```python
from build123d import *

# Parameters (mm, degrees)
EXTRUDE_1_DEPTH           = 60
CUT_EXTRUDE_1_DEPTH       = 423.965719651
CUT_EXTRUDE_1_DEPTH_BACK  = 25
HOLE_WIZARD_1_D           = 20
HOLE_WIZARD_1_CBORE_D     = 40
HOLE_WIZARD_1_CBORE_DEPTH = 20
EXTRUDE_START             = -32
EXTRUDE_3_DEPTH           = 72
CUT_EXTRUDE_3_DEPTH       = 531.913363931
CUT_EXTRUDE_3_DEPTH_BACK  = 531.913363931
SKETCH_10_R               = 40
SKETCH_12_R               = 80
CUT_EXTRUDE_5_DEPTH       = 20


with BuildPart() as part:
    # 草图1 → 凸台-拉伸1 (new body)
    with BuildSketch(Plane(origin=(0, 0, 0), x_dir=(1, 0, 0), z_dir=(0, 1, 0))):
        with BuildLine():
            Line((0, 0), (288, 0))
            ThreePointArc((288, 0), (310.627416998, -9.372583002), (320, -32))
            Line((320, -32), (320, -238))
            ThreePointArc((320, -238), (310.627416998, -260.627416998), (288, -270))
            Line((288, -270), (0, -270))
            Line((0, -270), (0, 0))
        make_face()
    extrude(amount=EXTRUDE_1_DEPTH)

    # 草图2 → 切除-拉伸1 (cut, two sides: drawn at the far end of the back side and taken through both)
    with BuildSketch(Plane.XZ.offset(-CUT_EXTRUDE_1_DEPTH_BACK)):
        with BuildLine():
            Line((230, 195), (320, 195))
            Line((320, 195), (320, 75))
            Line((320, 75), (230, 75))
            ThreePointArc((230, 75), (170, 135), (230, 195))
        make_face()
    extrude(amount=CUT_EXTRUDE_1_DEPTH + CUT_EXTRUDE_1_DEPTH_BACK, mode=Mode.SUBTRACT)

    # 孔1 (through all)
    with Locations(Plane(origin=(0, 60, 0), x_dir=(1, 0, 0), z_dir=(0, 1, 0))):
        with Locations((230, -135)):
            CounterBoreHole(HOLE_WIZARD_1_D / 2, HOLE_WIZARD_1_CBORE_D / 2, HOLE_WIZARD_1_CBORE_DEPTH)

    # 草图8 → 凸台-拉伸3 (add)
    with BuildSketch(Plane.ZY.offset(EXTRUDE_START)):
        with BuildLine():
            Line((0, 60), (270, 60))
            Line((270, 60), (270, 220))
            ThreePointArc((270, 220), (135, 355), (0, 220))
            Line((0, 220), (0, 60))
        make_face()
    extrude(amount=-EXTRUDE_3_DEPTH)

    # 草图10 → 切除-拉伸3 (cut, two sides: drawn at the far end of the back side and taken through both)
    with BuildSketch(Plane.ZY.offset(-32).offset(-CUT_EXTRUDE_3_DEPTH_BACK)):
        with Locations((135, 220)):
            Circle(SKETCH_10_R)
    extrude(amount=CUT_EXTRUDE_3_DEPTH + CUT_EXTRUDE_3_DEPTH_BACK, mode=Mode.SUBTRACT)

    # 草图12 → 切除-拉伸5 (cut)
    with BuildSketch(Plane.ZY.offset(-32)):
        with BuildLine():
            Line((255, 60), (255, 220))
            ThreePointArc((255, 220), (135, 340), (15, 220))
            Line((15, 220), (15, 60))
            Line((15, 60), (255, 60))
        make_face()
        with Locations((135, 220)):
            Circle(SKETCH_12_R, mode=Mode.SUBTRACT)
    extrude(amount=-CUT_EXTRUDE_5_DEPTH, mode=Mode.SUBTRACT)


solid = part.part
```
Could you check a few things on this model? Use its own coordinates, in mm. A direction names the side the tool comes from. Round coordinates to 2 decimals unless told otherwise and drop trailing zeros. Loops run counter-clockwise (first coordinate to the right, second up) from the corner with the lowest first, then second, coordinate; pieces in that order, holes last. Notation, with made-up numbers: (76.25, 27.25) -> (126.25, 27.25) arc R24 ccw to (126.25, 51.25) -> close; hole circle Ø1 at (25, -5.5). An arc over 180 degrees is marked (long way). Put each result on its own line as item: value.
Q1. I want a section at A-A on z = 135. Write out the boundary of the cut face in (x, y), and give its area (3 significant figures).
Checks:
outline: (0, 0) -> (170, 0) -> (170, 25) -> (220, 25) -> (220, 40) -> (210, 40) -> (210, 60) -> (104, 60) -> (104, 180) -> (32, 180) -> (32, 140) -> (52, 140) -> (52, 60) -> (0, 60) -> close; (32, 260) -> (104, 260) -> (104, 355) -> (32, 355) -> (32, 340) -> (52, 340) -> (52, 300) -> (32, 300) -> close; (240, 25) -> (320, 25) -> (320, 60) -> (250, 60) -> (250, 40) -> (240, 40) -> close
area: 27,400 mm2
Q2. Thinking about a two-plate mould opening in Y: for faces 5 (the cylindrical face through (67.496, 354.967, 137.969)), 6 (the cylindrical face through (170.015, 12.675, 133.681)), 7 (the cylindrical face through (41.86, 339.97, 137.64)), which applies, pulls with the +Y half, pulls with the -Y half, needs draft (parallel to the pull), parting line crosses it, or undercut?
Checks:
face 5: pulls with the +Y half
face 6: needs draft
face 7: undercut
Q3. For pin 1 Ø2 at (y, z) = (100.5, 223.5) entering from -X; pin 2 Ø1 at (x, z) = (124.5, 39.5) entering from +Y; pin 3 Ø6 at (x, z) = (214, 90) entering from -Y, each with a flat end and sliding along its axis, tell me the tip position at first contact or that it passes through.
Checks:
pin 1: x = 52
pin 2: y = 60
pin 3: y = 25
Q4. Which directions (+Z, -Z, +X, -X, +Y, -Y) give clear straight access to the entire face, cutting with the end or side of a thin tool? Please do faces 1 (the flat face through (274, 13, 195)), 2 (the cylindrical face through (41.86, 149.03, 171.92)), 3 (the cylindrical face through (214, 50, 147)), 4 (the flat face through (32, 230, 14)).
Checks:
face 1: +X, -Y
face 2: -X
face 3: +Y
face 4: +Z, -Z, -X, +Y
Q5. I want a section at D-D on z = 167.5. Write out the boundary of the cut face in (x, y), and give its area (3 significant figures).
Checks:
outline: (0, 0) -> (179.56, 0) -> (179.56, 25) -> (320, 25) -> (320, 60) -> (104, 60) -> (104, 196.68) -> (32, 196.68) -> (32, 146.9) -> (52, 146.9) -> (52, 60) -> (0, 60) -> close; (32, 243.32) -> (104, 243.32) -> (104, 351.03) -> (32, 351.03) -> (32, 335.52) -> (52, 335.52) -> (52, 293.1) -> (32, 293.1) -> close
area: 30,700 mm2
Q6. I want a section at B-B on y = 45.5. Write out the boundary of the cut face in (x, z), and give its area (3 significant figures).
Checks:
outline: (0, 0) -> (288, 0) arc R32 ccw to (320, 32) -> (320, 238) arc R32 ccw to (288, 270) -> (0, 270) -> close; hole circle Ø40 at (230, 135)
area: 84,700 mm2
Q7. Please list where these lines run through material, in increasing order: line 1 (Z direction, x = 230, y = 47); line 2 (Z direction, x = 55.5, y = 220); line 3 (Y direction, x = 74, z = 135). Write a range as from..to.
Checks:
line 1: 0..115, 155..270
line 2: 0..95, 175..270
line 3: 0..180, 260..355
Q8. I want a section at C-C on y = 252. Write out the boundary of the cut face in (x, z).
Checks:
outline: (32, 3.85) -> (104, 3.85) -> (104, 111) -> (32, 111) -> (32, 61.68) -> (52, 61.68) -> (52, 19.35) -> (32, 19.35) -> close; (32, 159) -> (104, 159) -> (104, 266.15) -> (32, 266.15) -> (32, 250.65) -> (52, 250.65) -> (52, 208.32) -> (32, 208.32) -> close
